Verification items for this drawing (mm, ordinates from the low corner). A direction names the side the tool comes from. Give positions to 0.01 mm unless a question says otherwise; leave off trailing zeros. Loops run counter-clockwise (first coordinate to the right, second up) from the corner with the lowest first, then second, coordinate; pieces in that order, holes last. Notation, with made-up numbers: M 3.25,77 L 20.25,77 A5 ccw 20.25,85 Z; hole C -2.5,41.25 d11. An arc over 180 degrees is marked long. Use a Markdown table: item, result.
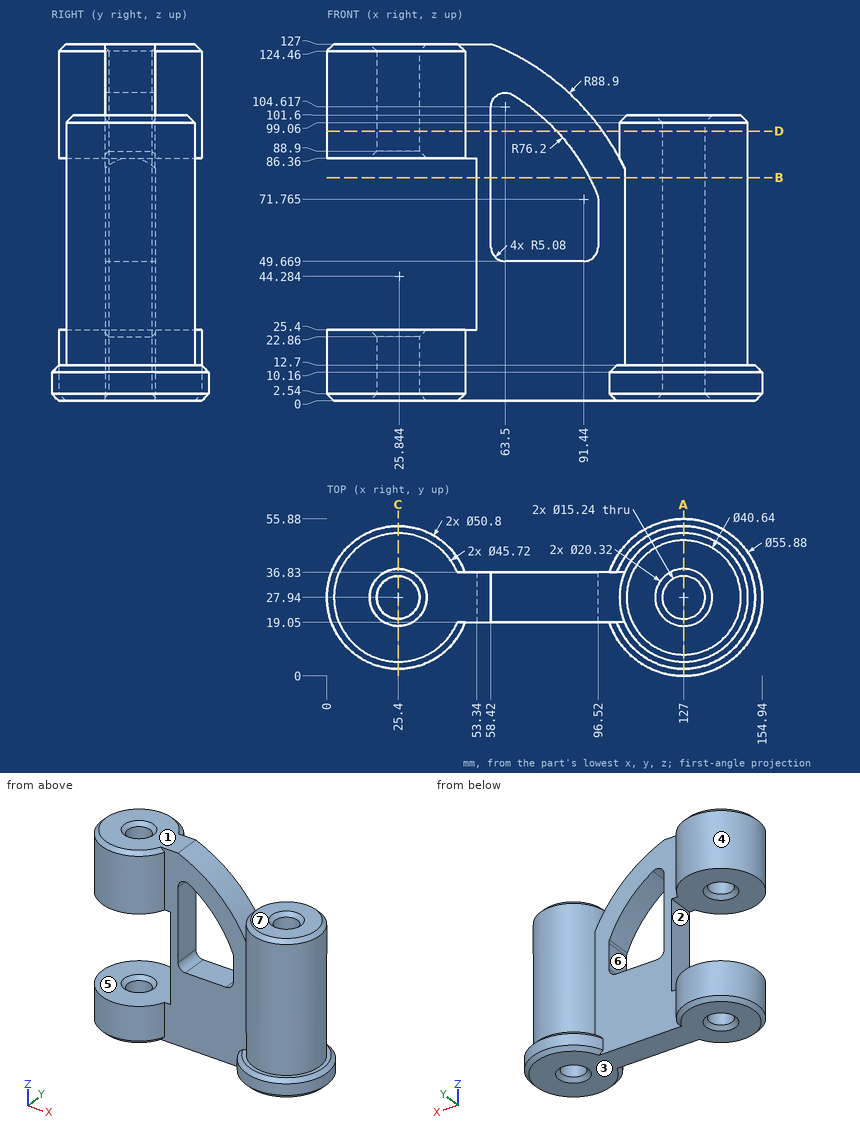
(1) Set-up check for the marked faces 4, 5, 6 and 7: record each of +Z, -Z, +X, -X, +Y, -Y from which the full face is reachable in a straight line by a thin tool's end or side.
Results below:
| item | result |
|---|---|
| face 4 | +Z, -Z |
| face 5 | -X, +Y, -Y |
| face 6 | +Y, -Y |
| face 7 | +Z, +X, +Y, -Y |
(2) Material ranges on line 1 (Y direction, x = 25.4, z = 104.5); line 2 (Y direction, x = 127, z = 35); line 3 (Z direction, x = 13.5, y = 38), recorded low to high.
Results below:
| item | result |
|---|---|
| line 1 | 2.54 to 20.32, 35.56 to 53.34 |
| line 2 | 5.08 to 20.32, 35.56 to 50.8 |
| line 3 | 0 to 25.4, 86.36 to 127 |
(3) Draft check along Z on the marked faces 1, 2 and 3. Enter one of: +Z half, -Z half, draft (parallel to the pull), parting line (faces both ways), or undercut.
Results below:
| item | result |
|---|---|
| face 1 | +Z half |
| face 2 | undercut |
| face 3 | -Z half |
(4) Gauge pin test, flat ends, axial feed: P1, Ø1.5, axis at y = 28, z = 37.5, coming from the +X side; P2, Ø20, axis at x = 127, y = 27.94, coming from the -Z side; P3, Ø9, axis at y = 27, z = 50.5, coming from the -X side. Record the tip position at first contact, or that the pin passes through.
Results below:
| item | result |
|---|---|
| P1 | x = 149.86 |
| P2 | z = 0.16 |
| P3 | x = 53.34 |
(5) Cross-section at A-A on x = 127. Record the cut outline in (y, z), then the cut area to 3 significant figures.
Results below:
| item | result |
|---|---|
| outline | M 0,2.54 L 2.54,0 L 17.78,0 L 20.32,2.54 L 20.32,99.06 L 17.78,101.6 L 7.62,101.6 L 5.08,99.06 L 5.08,12.7 L 2.54,12.7 L 0,10.16 Z; M 35.56,2.54 L 38.1,0 L 53.34,0 L 55.88,2.54 L 55.88,10.16 L 53.34,12.7 L 50.8,12.7 L 50.8,99.06 L 48.26,101.6 L 38.1,101.6 L 35.56,99.06 Z |
| area | 3,190 mm^2 |
(6) Cross-section at D-D on z = 96. Record the cut outline in (x, y), then the cut area to 3 significant figures.
Results below:
| item | result |
|---|---|
| outline | M 49.19,19.05 L 58.42,19.05 L 58.42,36.83 L 49.19,36.83 A25.4 ccw long Z; M 81.81,19.05 L 98.15,19.05 L 98.15,36.83 L 81.81,36.83 Z; C 127,27.94 d45.72; hole C 25.4,27.94 d15.24; hole C 127,27.94 d15.24 |
| area | 3,740 mm^2 |
(7) Cross-section at B-B on z = 79.5. Record the cut outline in (x, y), then the cut area to 3 significant figures.
Results below:
| item | result |
|---|---|
| outline | M 53.34,19.05 L 58.42,19.05 L 58.42,36.83 L 53.34,36.83 Z; M 93.42,19.05 L 105.94,19.05 A22.86 ccw long 105.94,36.83 L 93.42,36.83 Z; hole C 127,27.94 d15.24 |
| area | 1,750 mm^2 |
(8) Cross-section at C-C on x = 25.4. Record the cut outline in (y, z), then the cut area to 3 significant figures.
Results below:
| item | result |
|---|---|
| outline | M 2.54,2.54 L 5.08,0 L 17.78,0 L 20.32,2.54 L 20.32,22.86 L 17.78,25.4 L 2.54,25.4 Z; M 2.54,86.36 L 17.78,86.36 L 20.32,88.9 L 20.32,124.46 L 17.78,127 L 5.08,127 L 2.54,124.46 Z; M 35.56,2.54 L 38.1,0 L 50.8,0 L 53.34,2.54 L 53.34,25.4 L 38.1,25.4 L 35.56,22.86 Z; M 35.56,88.9 L 38.1,86.36 L 53.34,86.36 L 53.34,124.46 L 50.8,127 L 38.1,127 L 35.56,124.46 Z |
| area | 2,310 mm^2 |
